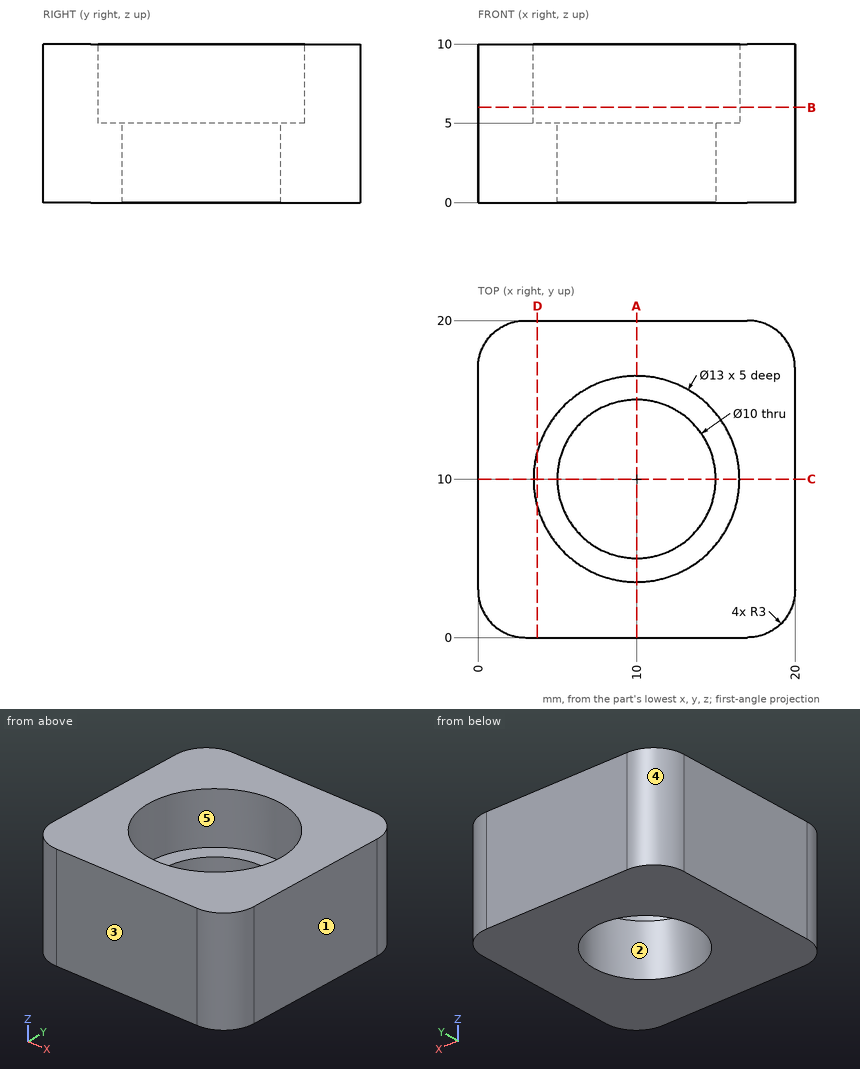
For this review, use the dimensioned drawing (mm, ordinates from the lowest corner) and the shaded views. A direction names the side the tool comes from. Round coordinates to 2 decimals unless told otherwise and drop trailing zeros. Order: outer loops, then holes, each group sorted by start corner. A loop starts at its lowest first (then second) coordinate and runs counter-clockwise, first axis right, second up. Notation, with made-up numbers: (-31.75, -31) -> (13.25, -31) arc R6 ccw to (13.25, -23) -> close; hole circle Ø10 at (-23, -35). An arc over 180 degrees is marked (long way). Use CSV: the item, a comma, the result in double quotes. Start each with the question number.
(1) Mouldability with a two-part tool opening along X and no side actions: class the marked faces 1, 2 and 3 as pulls with the +X half, pulls with the -X half, needs draft (parallel to the pull), parting line crosses it, or undercut.
(2) Insertion check: pin 1 (11.5 mm diameter, centred on x = 10, y = 10, fed in from +Z); pin 2 (6 mm diameter, centred on x = 3, y = 3.5, fed in from -Z). Each pin has a flat end and moves straight along its axis. Give the tip position at first contact, or say it passes through.
(3) Tool access review of the marked faces 4 and 5: name each direction out of +Z, -Z, +X, -X, +Y, -Y from which nothing blocks a thin tool from reaching the whole face with its end or side.
(4) Wall thickness on probe 1 along Y at (x, z) = (10, 3.2); probe 2 along Y at (x, z) = (10, 6.65); probe 3 along Z at (x, y) = (5, 7): over which ranges is each line inside the solid? List them lowest first. Write a range as from..to.
(5) Consider section D-D on x = 3.75. Write out the cut boundary in (y, z), and give its area (3 significant figures).
(6) Consider section B-B on z = 6. Write out the cut boundary in (x, y).
(7) Consider section A-A on x = 10. Write out the cut boundary in (y, z), and give its area (3 significant figures).
Responses:
1,face 1,"pulls with the +X half"
1,face 2,"undercut"
1,face 3,"needs draft"
2,pin 1,"z = 5"
2,pin 2,"z = 0"
3,face 4,"+Z, -Z, -X, +Y"
3,face 5,"+Z"
4,probe 1,"0..5, 15..20"
4,probe 2,"0..3.5, 16.5..20"
4,probe 3,"0..5"
5,outline,"(0, 0) -> (20, 0) -> (20, 10) -> (11.79, 10) -> (11.79, 5) -> (8.21, 5) -> (8.21, 10) -> (0, 10) -> close"
5,area,"182 mm²"
6,outline,"(0, 3) arc R3 ccw to (3, 0) -> (17, 0) arc R3 ccw to (20, 3) -> (20, 17) arc R3 ccw to (17, 20) -> (3, 20) arc R3 ccw to (0, 17) -> close; hole circle Ø13 at (10, 10)"
7,outline,"(0, 0) -> (5, 0) -> (5, 5) -> (3.5, 5) -> (3.5, 10) -> (0, 10) -> close; (15, 0) -> (20, 0) -> (20, 10) -> (16.5, 10) -> (16.5, 5) -> (15, 5) -> close"
7,area,"85.0 mm²"
